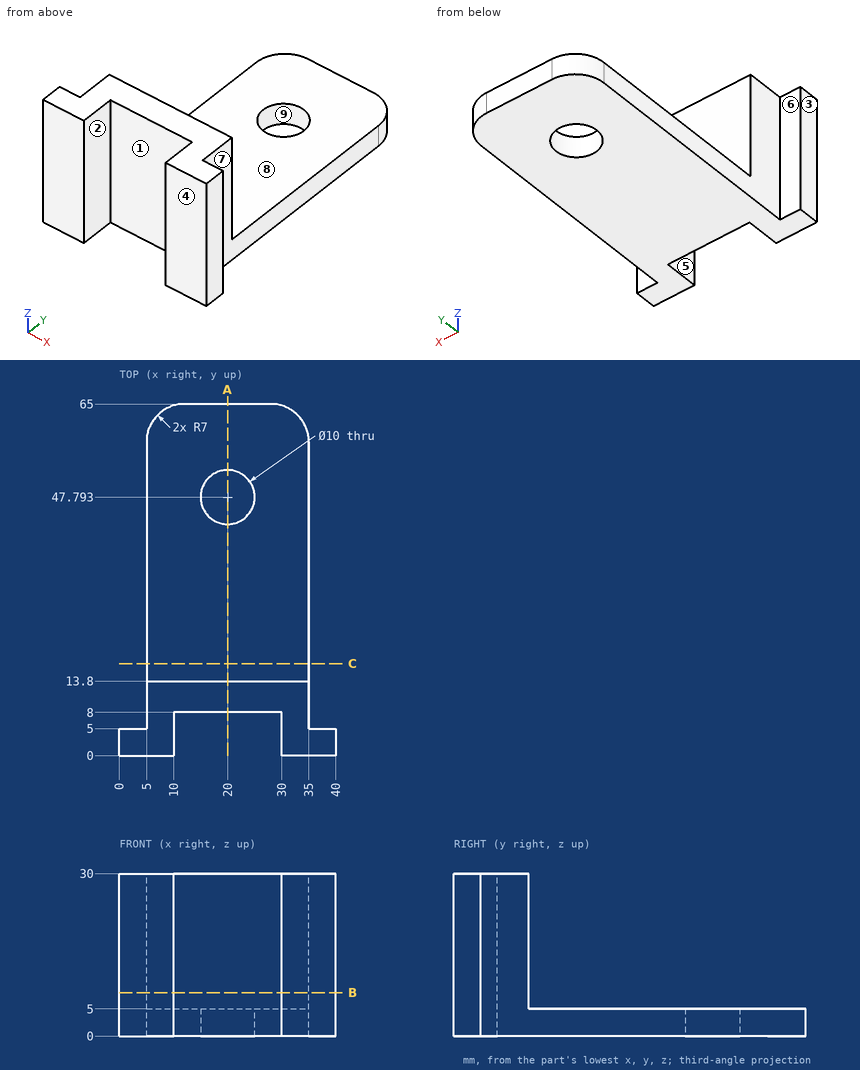
Source: three-view drawing plus pictorial views. Frame: mm from the lowest corner of the part. A direction names the side the tool comes from. Coordinates: 2 decimals unless noted, no trailing zeros. Order: outer loops, then holes, each group sorted by start corner. A loop starts at its lowest first (then second) coordinate and runs counter-clockwise, first axis right, second up. Notation, with made-up numbers: M 53,48 L 57,48 A20 ccw 57,78 Z; hole C 41,-38.75 d11. An arc over 180 degrees is marked long. Answer in a Markdown table with one row per item.
(1) Material intervals for line 1 (Y direction, x = 20, z = 3); line 2 (Y direction, x = 17.5, z = 26); line 3 (X direction, y = 11, z = 7.5), sorted ascending. Write a range as [from, to].
Numbers:
| item | result |
|---|---|
| line 1 | y = [8, 42.79], [52.79, 65] |
| line 2 | y = [8, 13.8] |
| line 3 | x = [5, 35] |
(2) Section query B-B, the plane z = 8. Output: boundary loops of the cut face in (x, y), plus the area to 3 significant figures.
Numbers:
| item | result |
|---|---|
| outline | M 0,0 L 10,0 L 10,8 L 30,8 L 30,0 L 40,0 L 40,5 L 35,5 L 35,13.8 L 5,13.8 L 5,5 L 0,5 Z |
| area | 304 mm^2 |
(3) Access query for the marked faces 5, 6, 7, 8 and 9. Directions: +Z, -Z, +X, -X, +Y, -Y. A direction counts if a zero-diameter tool reaches every point of the face in a straight line with its end or side. Return the directions, or none.
Numbers:
| item | result |
|---|---|
| face 5 | +Z, -Z, -Y |
| face 6 | +Z, -Z, -X, +Y |
| face 7 | +Z, -Z, +X, +Y |
| face 8 | +Z, +X, -X, +Y |
| face 9 | +Z, -Z |
(4) Section query A-A, the plane x = 20. Output: boundary loops of the cut face in (y, z), plus the area to 3 significant figures.
Numbers:
| item | result |
|---|---|
| outline | M 8,0 L 42.79,0 L 42.79,5 L 13.8,5 L 13.8,30 L 8,30 Z; M 52.79,0 L 65,0 L 65,5 L 52.79,5 Z |
| area | 380 mm^2 |
(5) Section query C-C, the plane y = 17. Output: boundary loops of the cut face in (x, z).
Numbers:
| item | result |
|---|---|
| outline | M 5,0 L 35,0 L 35,5 L 5,5 Z |
(6) Draft query along X for the marked faces 1, 2, 3 and 4. Return one class per face: pulls with the +X half, pulls with the -X half, needs draft (parallel to the pull), parting line crosses it, or undercut.
Numbers:
| item | result |
|---|---|
| face 1 | undercut |
| face 2 | undercut |
| face 3 | pulls with the -X half |
| face 4 | needs draft |
(7) Contact query for flat-ended pins moving along their axis: pin 1 Ø1.5 at (x, z) = (38.5, 21.5) entering from +Y; pin 2 Ø1.5 at (x, z) = (26.5, 20) entering from +Y; pin 3 Ø15 at (y, z) = (23, 12) entering from -X; pin 4 Ø16 at (x, z) = (22.5, 9.5) entering from -Y. Output: stop coordinate, or through.
Numbers:
| item | result |
|---|---|
| pin 1 | stops at y = 5 |
| pin 2 | stops at y = 13.8 |
| pin 3 | stops at x = 5 |
| pin 4 | stops at y = 0 |
